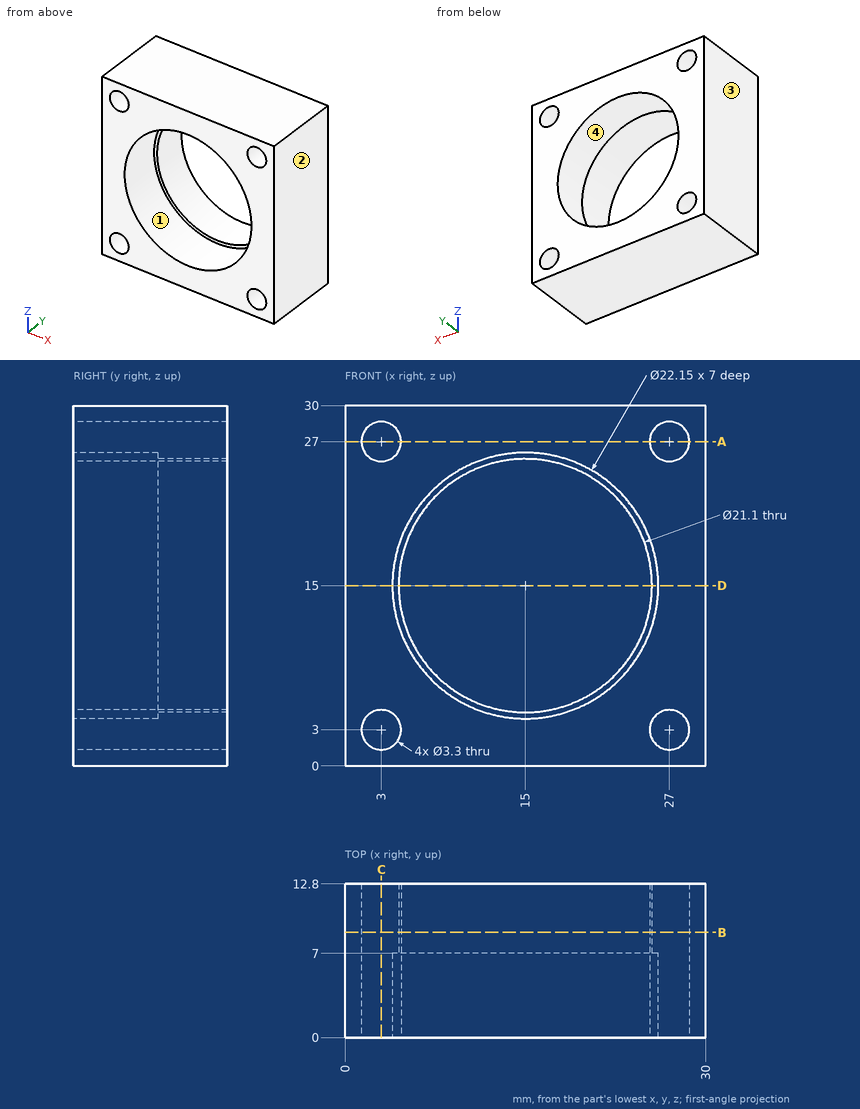
Geometry: see drawing. Coordinates: mm, zero at the bounding-box minimum. Round coordinates to 2 decimals unless told otherwise and drop trailing zeros. Write each loop counter-clockwise with the first axis right and the second up, starting at its lowest first coordinate (ties: lowest second). Pieces come first, ordered by that corner, then holes. Notation, with made-up numbers: M -8,30 L 21,30 A9 ccw 21,44 Z; hole C -11,29.25 d9. An arc over 180 degrees is marked long. Answer as a JSON object with one key per item and string values. Group by question number.
(1) Mould query, pull axis X, two halves, no side actions, for the marked faces 1, 2, 3 and 4. Classes: +X half, -X half, draft (parallel to the pull), parting line (faces both ways), or undercut.
(2) Section query B-B on y = 8.75. Output: boundary loops of the cut face in (x, z), then the cut area to 3 significant figures.
(3) First-contact query: pin 1 (4.5 mm diameter, centred on x = 3, z = 3, fed in from -Y). Flat tip, straight axial feed; report the tip coordinate or a pass-through.
(4) Section query C-C on x = 3. Output: boundary loops of the cut face in (y, z), then the cut area to 3 significant figures.
(5) Section query A-A on z = 27. Output: boundary loops of the cut face in (x, y).
(6) Ray query, line 1 (Z direction, x = 27, y = 9.5); line 2 (Z direction, x = 15, y = 8.45). Return the intervals inside material, ascending. Write a range as [from, to].
(7) Section query D-D on z = 15. Output: boundary loops of the cut face in (x, y) (3 decimals), then the cut area to 3 significant figures.
Computed values:
{
 "1": {"face 1": "undercut", "face 2": "+X half", "face 3": "-X half", "face 4": "undercut"},
 "2": {"outline": "M 0,0 L 30,0 L 30,30 L 0,30 Z; hole C 3,3 d3.3; hole C 3,27 d3.3; hole C 15,15 d21.1; hole C 27,3 d3.3; hole C 27,27 d3.3", "area": "516 mm^2"},
 "3": {"pin 1": "y = 0"},
 "4": {"outline": "M 0,0 L 12.8,0 L 12.8,1.35 L 0,1.35 Z; M 0,4.65 L 12.8,4.65 L 12.8,25.35 L 0,25.35 Z; M 0,28.65 L 12.8,28.65 L 12.8,30 L 0,30 Z", "area": "300 mm^2"},
 "5": {"outline": "M 0,0 L 1.35,0 L 1.35,12.8 L 0,12.8 Z; M 4.65,0 L 25.35,0 L 25.35,12.8 L 4.65,12.8 Z; M 28.65,0 L 30,0 L 30,12.8 L 28.65,12.8 Z"},
 "6": {"line 1": "[0, 1.35], [4.65, 25.35], [28.65, 30]", "line 2": "[0, 4.45], [25.55, 30]"},
 "7": {"outline": "M 0,0 L 3.925,0 L 3.925,7 L 4.45,7 L 4.45,12.8 L 0,12.8 Z; M 25.55,7 L 26.075,7 L 26.075,0 L 30,0 L 30,12.8 L 25.55,12.8 Z", "area": "107 mm^2"}
}
